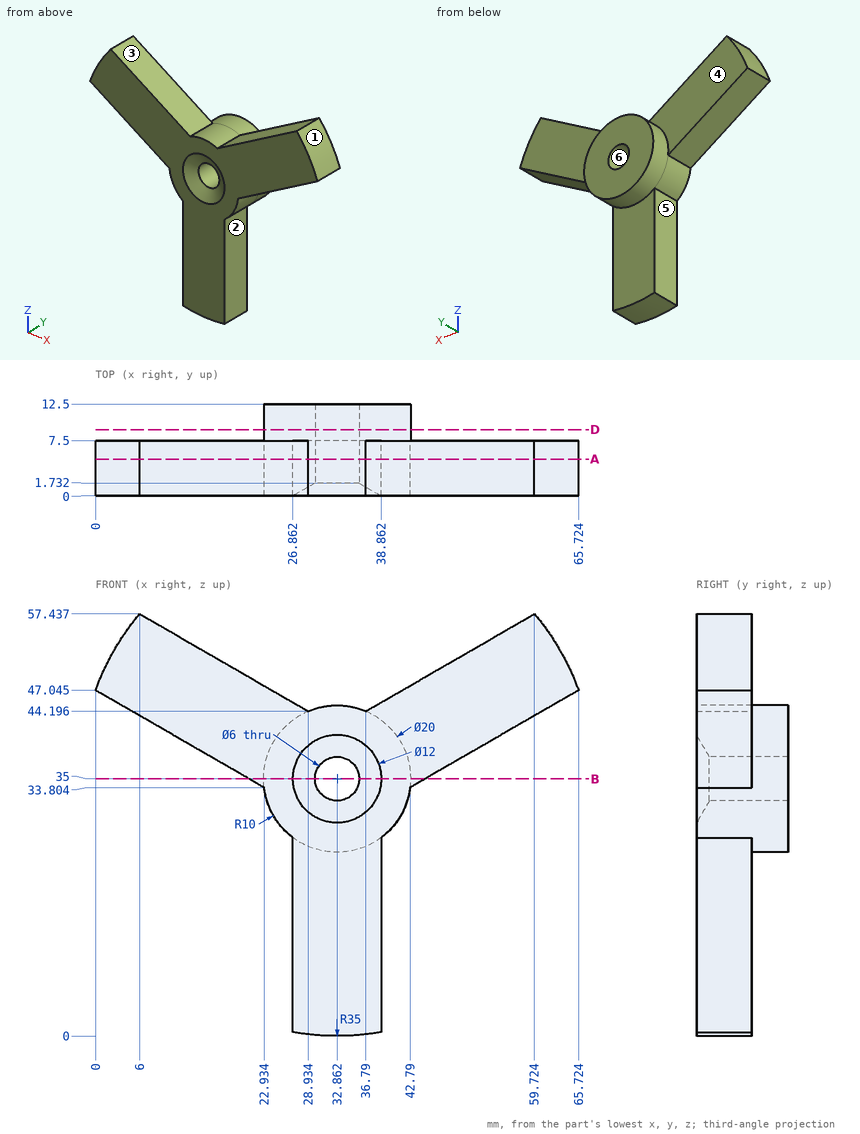
Geometry check sheet. Reference: drawing and pictorial views, mm from the part's lowest x, y, z. A direction names the side the tool comes from. Round coordinates to 2 decimals unless told otherwise and drop trailing zeros. Order: outer loops, then holes, each group sorted by start corner. A loop starts at its lowest first (then second) coordinate and runs counter-clockwise, first axis right, second up. Notation, with made-up numbers: M 25.5,-35.75 L 69.5,-35.75 A13 ccw 69.5,-28.75 Z; hole C 78.25,86 d8. An arc over 180 degrees is marked long. Answer as CSV lines item,"result".
1) Gauge pin test, flat ends, axial feed: pin 1 Ø7 at (x, z) = (32.86, 35) entering from -Y; pin 2 Ø7 at (x, z) = (11, 48.5) entering from +Y; pin 3 Ø5 at (y, z) = (4.5, 44.5) entering from +X (1 decimal). Record the tip position at first contact, or that the pin passes through.
Entries:
pin 1,"y = 1.44"
pin 2,"y = 7.5"
pin 3,"x = 65.6"
2) Sectioned sample at A-A on y = 5. Record the cut outline in (x, z) (1 decimal), and give its area (3 significant figures).
Entries:
outline,"M 0,47 L 22.9,33.8 A10 ccw 26.9,27 L 26.9,0.5 A35 ccw 38.9,0.5 L 38.9,27 A10 ccw 42.8,33.8 L 65.7,47 A35 ccw 59.7,57.4 L 36.8,44.2 A10 ccw 28.9,44.2 L 6,57.4 A35 ccw Z; hole C 32.9,35 d6"
area,"1,200 mm2"
3) Tool access check on the marked faces 1 and 2. Record the directions out of +Z, -Z, +X, -X, +Y, -Y that give a thin tool (end or side, any length) a straight path to the whole face; none if there is none.
Entries:
face 1,"+Z, +X, +Y, -Y"
face 2,"-Z, +X, +Y, -Y"
4) Mould release check, pull along X, two halves, no side actions. Record for the marked faces 3, 4, 5 and 6: +X half, -X half, draft (parallel to the pull), parting line (faces both ways), or undercut.
Entries:
face 3,"undercut"
face 4,"draft"
face 5,"-X half"
face 6,"undercut"
5) Sectioned sample at B-B on z = 35. Record the cut outline in (x, y), and give its area (3 significant figures).
Entries:
outline,"M 20.86,0 L 26.86,0 L 29.86,1.73 L 29.86,12.5 L 22.86,12.5 L 22.86,7.5 L 20.86,7.5 Z; M 35.86,1.73 L 38.86,0 L 44.86,0 L 44.86,7.5 L 42.86,7.5 L 42.86,12.5 L 35.86,12.5 Z"
area,"200 mm2"
6) Thickness scan on probe 1 along X at (y, z) = (9, 35); probe 2 along Y at (x, z) = (19, 39); probe 3 along X at (y, z) = (5.5, 9). Record the ranges inside material, lowest first. Write a range as [from, to].
Entries:
probe 1,"[22.86, 29.86], [35.86, 42.86]"
probe 2,"[0, 7.5]"
probe 3,"[26.86, 38.86]"
7) Sectioned sample at D-D on y = 9. Record the cut outline in (x, z), and give its area (3 significant figures).
Entries:
outline,"C 32.86,35 d20; hole C 32.86,35 d6"
area,"286 mm2"
